from build123d import *

# Parameters (mm, degrees)
F0_R     = 9
F1_DEPTH = 20.5
F2_R     = 6
F3_DEPTH = 16.5
F4_R     = 3
F5_DEPTH = 17.5


with BuildPart() as f1:
    # F0 (on Top) → F1 (new body)
    with BuildSketch(Plane.XY):
        Circle(F0_R)
    extrude(amount=F1_DEPTH)

    # F2 (on Top) → F3 (cut)
    with BuildSketch(Plane.XY):
        Circle(F2_R)
    extrude(amount=F3_DEPTH, mode=Mode.SUBTRACT)

    # F4 (on Top) → F5 (cut)
    with BuildSketch(Plane.XY):
        Circle(F4_R)
    extrude(amount=F5_DEPTH, mode=Mode.SUBTRACT)


solid = f1.part
Read the model definition and answer for the solid it produces. Units are mm, in the model's axes. A direction names the side the tool comes from. Give positions to 0.01 mm unless a question says otherwise; leave off trailing zeros. Loops run counter-clockwise (first coordinate to the right, second up) from the corner with the lowest first, then second, coordinate; pieces in that order, holes last. Notation, with made-up numbers: (21, -29.5) - (61, -29.5) arc R33 cw to (61, 8.5) - close; hole circle Ø11 at (22, 70). An arc over 180 degrees is marked (long way). Answer as CSV lines item,"result". Start each with the question number.
1) Find section D-D (y = 7.75). Write down the section's boundary in (x, z), then the cut area to 3 significant figures.
2) Each of these flat-tipped pins is pushed along its axis until it touches: pin 1 Ø6 at (y, z) = (4.5, 14) entering from +X; pin 2 Ø3.5 at (x, y) = (-2.5, -0.5) entering from -Z; pin 3 Ø8 at (y, z) = (-6.5, 14.5) entering from +X. Where does it stop, or does it pass through?
3) Find section C-C (x = -4.75). Write down the section's boundary in (y, z).
4) Determine the mould class of faces 1 (the face through (2, -6, 0)), 2 (the face through (-3, 0, 17)), 3 (the face through (-3, -1, 16.5)), 4 (the face through (-1.172, 8.923, 10.106)) for opening direction X: released by +X, released by -X, zero draft, split by the parting line, or undercut.
5) Find section A-A (y = 0). Write down the section's boundary in (x, z).
6) Which of the six approach directions +Z, -Z, +X, -X, +Y, -Y give full straight-line access (tool end or side, diameter ignored) to faces 5 (the face through (0, 0, 20.5)), 6 (the face through (0, 0, 17.5))?
7) Find section B-B (x = 2.5). Write down the section's boundary in (y, z), then the cut area to 3 significant figures.
8) Straight lines are drawn through the part: L1, parallel to Y at x = 0, z = 16.7; L2, parallel to Y at x = 0, z = 12.25; L3, parallel to Z at x = 1.25, y = -0.75. For each, find the intervals that lie inside material, in ascending order. Write a range as from..to.
Findings below:
1,outline,"(-4.58, 0) - (4.58, 0) - (4.58, 20.5) - (-4.58, 20.5) - close"
1,area,"188 mm^2"
2,pin 1,"x = 8.87"
2,pin 2,"z = 16.5"
2,pin 3,"x = 8.65"
3,outline,"(-7.64, 0) - (-3.67, 0) - (-3.67, 16.5) - (3.67, 16.5) - (3.67, 0) - (7.64, 0) - (7.64, 20.5) - (-7.64, 20.5) - close"
4,face 1,"zero draft"
4,face 2,"undercut"
4,face 3,"undercut"
4,face 4,"split by the parting line"
5,outline,"(-9, 0) - (-6, 0) - (-6, 16.5) - (-3, 16.5) - (-3, 17.5) - (3, 17.5) - (3, 16.5) - (6, 16.5) - (6, 0) - (9, 0) - (9, 20.5) - (-9, 20.5) - close"
6,face 5,"+Z, +X, -X, +Y, -Y"
6,face 6,"-Z"
7,outline,"(-8.65, 0) - (-5.45, 0) - (-5.45, 16.5) - (-1.66, 16.5) - (-1.66, 17.5) - (1.66, 17.5) - (1.66, 16.5) - (5.45, 16.5) - (5.45, 0) - (8.65, 0) - (8.65, 20.5) - (-8.65, 20.5) - close"
7,area,"171 mm^2"
8,L1,"-9..-3, 3..9"
8,L2,"-9..-6, 6..9"
8,L3,"17.5..20.5"
